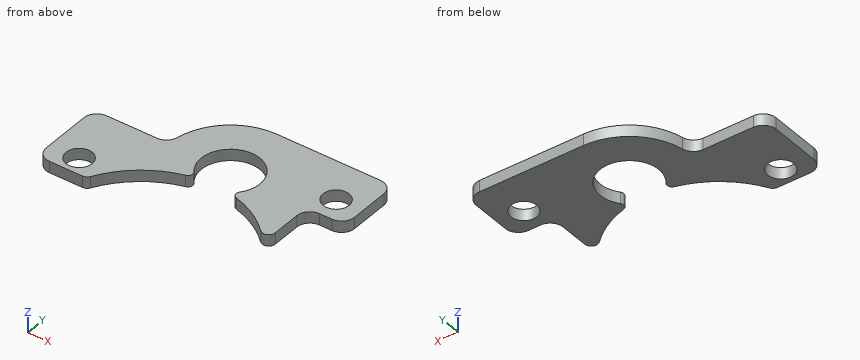
```python
from build123d import *

# Parameters (mm, degrees)
SKETCH1_R           = 2
BOSS_EXTRUDE2_DEPTH = 1.75


with BuildPart() as part:
    # Sketch1 → Boss-Extrude2 (new body)
    with BuildSketch(Plane.XY):
        with BuildLine():
            Line((0, 9.5), (15.95, 9.5))
            ThreePointArc((15.95, 9.5), (17.364213562, 8.914213562), (17.95, 7.5))
            Line((17.95, 7.5), (17.95, 1.5))
            ThreePointArc((17.95, 1.5), (17.364213562, 0.085786438), (15.95, -0.5))
            Line((15.95, -0.5), (14.05, -0.5))
            ThreePointArc((14.05, -0.5), (12.635786438, -1.085786438), (12.05, -2.5))
            Line((12.05, -2.5), (12.05, -2.621320344))
            Line((12.05, -2.621320344), (12.05, -6.92859127))
            ThreePointArc((12.05, -6.92859127), (11.443303318, -7.848000047), (10.359375, -7.651804315))
            ThreePointArc((10.359375, -7.651804315), (7.356020854, -5.427549686), (3.896023084, -4.014800515))
            ThreePointArc((3.896023084, -4.014800515), (3.377802295, -3.523133979), (3.506420776, -2.82046332))
            ThreePointArc((3.506420776, -2.82046332), (4.482227913, -0.399540902), (3.95, 2.155806114))
            ThreePointArc((3.95, 2.155806114), (-2.498000201, 3.742992786), (-3.506420776, -2.82046332))
            ThreePointArc((-3.506420776, -2.82046332), (-3.377802295, -3.523133979), (-3.896023084, -4.014800515))
            ThreePointArc((-3.896023084, -4.014800515), (-9.243460442, -6.686514525), (-13.122907199, -11.234375))
            ThreePointArc((-13.122907199, -11.234375), (-13.490015279, -11.611503047), (-13.997767679, -11.75))
            Line((-13.997767679, -11.75), (-19.05, -11.75))
            ThreePointArc((-19.05, -11.75), (-20.464213562, -11.164213562), (-21.05, -9.75))
            Line((-21.05, -9.75), (-21.05, -2))
            ThreePointArc((-21.05, -2), (-20.464213562, -0.585786438), (-19.05, 0))
            Line((-19.05, 0), (-11.324751653, 0))
            ThreePointArc((-11.324751653, 0), (-10.039382479, 0.467738245), (-9.355229626, 1.652173913))
            ThreePointArc((-9.355229626, 1.652173913), (-6.105503576, 7.278243338), (0, 9.5))
        make_face()
        with Locations((-16.55, -9)):
            Circle(SKETCH1_R, mode=Mode.SUBTRACT)
        with Locations((13.95, 3.05)):
            Circle(SKETCH1_R, mode=Mode.SUBTRACT)
    extrude(amount=BOSS_EXTRUDE2_DEPTH)


solid = part.part
```
Here's how the part is built. I have some questions about the finished solid (model axes, mm). Coordinates: 2 decimals unless noted, no trailing zeros. Order: outer loops, then holes, each group sorted by start corner. A loop starts at its lowest first (then second) coordinate and runs counter-clockwise, first axis right, second up.
1) Imagine slicing it at D-D on x = -18. List the corners of the cut face in (y, z) for me, and give its area (3 significant figures).
2) Imagine slicing it at A-A on y = 3.05. List the corners of the cut face in (x, z) for me.
3) Imagine slicing it at B-B on y = -9. List the corners of the cut face in (x, z) for me, and give its area (3 significant figures).
4) I need wall thicknesses on line 1 (Y direction, x = -16.55, z = 1.3); line 2 (Y direction, x = 13.95, z = 0.9); line 3 (X direction, y = -3.5, z = 0.85). Which ranges of each line are inside material? Lowest first, please.
5) Will these pins go through, and if not, where does the flat tip stop? pin 1 (0.9 mm diameter, centred on x = 14.5, z = 1, fed in from -Y); pin 2 (5 mm diameter, centred on x = 13.95, y = 3.05, fed in from +Z); pin 3 (8 mm diameter, centred on x = 0, y = 0, fed in from -Z); pin 4 (1 mm diameter, centred on y = 6.5, z = 0.5, fed in from -X).
6) Imagine slicing it at C-C on z = 1.3. List the corners of the cut face in (x, y) for me, and give its area (3 significant figures).
Response values:
1. outline: (-11.75, 0) - (-10.38, 0) - (-10.38, 1.75) - (-11.75, 1.75) - close; (-7.62, 0) - (0, 0) - (0, 1.75) - (-7.62, 1.75) - close
1. area: 15.7 mm2
2. outline: (-9, 0) - (-3.31, 0) - (-3.31, 1.75) - (-9, 1.75) - close; (3.31, 0) - (11.95, 0) - (11.95, 1.75) - (3.31, 1.75) - close; (15.95, 0) - (17.95, 0) - (17.95, 1.75) - (15.95, 1.75) - close
3. outline: (-21.05, 0) - (-18.55, 0) - (-18.55, 1.75) - (-21.05, 1.75) - close; (-14.55, 0) - (-11.61, 0) - (-11.61, 1.75) - (-14.55, 1.75) - close
3. area: 9.52 mm2
4. line 1: y = -11.75 to -11, -7 to 0
4. line 2: y = -0.5 to 1.05, 5.05 to 9.5
4. line 3: x = -21.05 to -3.37, 3.37 to 12.05
5. pin 1: stops at y = -0.5
5. pin 2: stops at z = 1.75
5. pin 3: passes through
5. pin 4: stops at x = -7.37
6. outline: (-21.05, -9.75) arc R2 ccw to (-19.05, -11.75) - (-14, -11.75) arc R1 ccw to (-13.12, -11.23) arc R15 cw to (-3.9, -4.01) arc R0.75 ccw to (-3.51, -2.82) arc R4.5 cw (long way) to (3.51, -2.82) arc R0.75 ccw to (3.9, -4.01) arc R15 cw to (10.36, -7.65) arc R1 ccw to (12.05, -6.93) - (12.05, -2.5) arc R2 cw to (14.05, -0.5) - (15.95, -0.5) arc R2 ccw to (17.95, 1.5) - (17.95, 7.5) arc R2 ccw to (15.95, 9.5) - (0, 9.5) arc R9.5 ccw to (-9.36, 1.65) arc R2 cw to (-11.32, 0) - (-19.05, 0) arc R2 ccw to (-21.05, -2) - close; hole circle Ø4 at (-16.55, -9); hole circle Ø4 at (13.95, 3.05)
6. area: 387 mm2
